Autodesk Inventor part; units mm, degrees
ref_plane "YZ Plane" through (0, 0, 0) normal (1, 0, 0) x (0, 1, 0)
ref_plane "XZ Plane" through (0, 0, 0) normal (0, 1, 0) x (-1, 0, 0)
ref_plane "XY Plane" through (0, 0, 0) normal (0, 0, 1) x (1, 0, 0)
sketch "Sketch1" plane through (0, 0, 0) normal (0, 1, 0) x (-1, 0, 0)
  circle A0 centre (-65.9389, 138.5386) radius 14
  circle A1 centre (-65.9389, 138.5386) radius 13.746
  circle A2 centre (-65.9389, 138.5386) radius 31.75
  point P0 (0, 0)
  dimension "d0" = 27.492
  dimension "d1" = 28
  dimension "d2" = 63.5
extrude "Extrusion1" add sketch "Sketch1" along normal blind 3.175 contours A0 | A1 | A2
sketch "Sketch2" plane through (65.9389, 0, 138.5386) normal (0, -1, 0) x (1, 0, 0)
  circle A0 centre (0, 0) radius 13.746
  point P0 (-65.9389, -138.5386)
  dimension "d5" = 27.492
extrude "Extrusion2" add sketch "Sketch2" along normal blind 38.1
sketch "Sketch3" plane through (65.9389, 0, 138.5386) normal (0, -1, 0) x (1, 0, 0)
  circle A0 centre (0, 23.8125) radius 2.1526
  circle A1 centre (20.6222, 11.9062) radius 2.1526
  circle A2 centre (20.6222, -11.9063) radius 2.1526
  circle A3 centre (0, -23.8125) radius 2.1526
  circle A4 centre (-20.6222, -11.9062) radius 2.1526
  circle A5 centre (-20.6222, 11.9063) radius 2.1526
  circle A6 centre (0, 23.8125) radius 1.8986
  circle A7 centre (20.6222, 11.9062) radius 1.8986
  circle A8 centre (20.6222, -11.9063) radius 1.8986
  circle A9 centre (-20.6222, -11.9062) radius 1.8986
  circle A10 centre (-20.6222, 11.9063) radius 1.8986
  circle A11 centre (0, -23.8125) radius 1.8986
  point P0 (-65.9389, -138.5386)
  dimension "d8" = 4.3053
  dimension "d9" = 3.7973
  dimension "d10" = 3.7973
  dimension "d11" = 3.7973
  dimension "d12" = 3.7973
  dimension "d13" = 3.7973
  dimension "d14" = 3.7973
extrude "Extrusion3" add sketch "Sketch3" along normal blind 12.7 contours A6 | A7 | A8 | A9 | A10 | A11
properties part number "5inCompliantWheelHub"
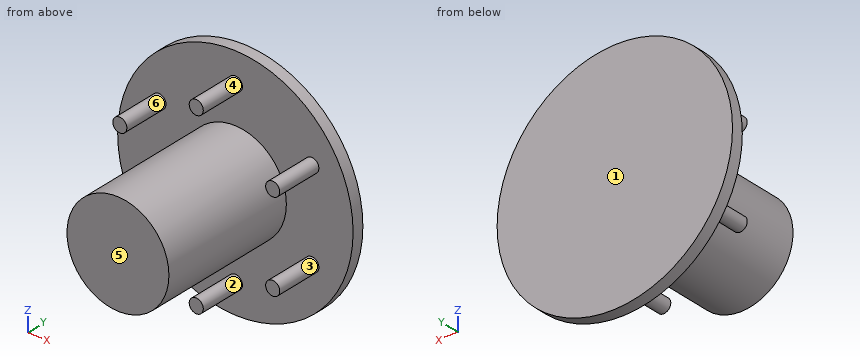
Can you work these out from the model? Positions are in its coordinate system, mm. Face numbers are marked on the shaded views. A direction names the side the tool comes from. Round coordinates to 2 decimals unless told otherwise and drop trailing zeros. Order: outer loops, then holes, each group sorted by start corner. A loop starts at its lowest first (then second) coordinate and runs counter-clockwise, first axis right, second up. Notation, with made-up numbers: (64, 35) -> (74, 35) arc R21 cw to (74, 45) -> close; hole circle Ø1 at (9, 78). An arc over 180 degrees is marked (long way). Return JSON: item names as keys, results as strings. Group by question number.
1. Will these pins go through, and if not, where does the flat tip stop? pin 1 (1.1 mm diameter, centred on x = 85.5, z = 151, fed in from -Y); pin 2 (1.5 mm diameter, centred on y = -15, z = 136, fed in from +X); pin 3 (2 mm diameter, centred on x = 79, z = 158, fed in from -Y).
2. We'd pull the mould along X, two halves only. Please class the marked faces 3, 4, 5 and 6: released by +X, released by -X, zero draft, split by the parting line, or undercut.
3. I need wall thicknesses on line 1 (Z direction, x = 45.5, y = -7.5); line 2 (Y direction, x = 68, z = 117.5) (3 decimals); line 3 (X direction, y = -9, z = 131). Which ranges of each line are inside material? Lowest first, please. Write a range as [from, to].
4. Which directions (+Z, -Z, +X, -X, +Y, -Y) give clear straight access to the entire face, cutting with the end or side of a thin tool? Please do the marked faces 1 and 2.
5. If we section it at C-C, the plane z = 144: Write out the boundary of the cut face in (x, y) (3 decimals), then the cut area to 3 significant figures.
6. If we section it at B-B, the plane x = 70: Write out the boundary of the cut face in (y, z) (3 decimals).
7. If we section it at D-D, the plane y = -22: Write out the boundary of the cut face in (x, z), then the cut area to 3 significant figures.
8. If we section it at A-A, the plane y = -3: Write out the boundary of the cut face in (x, z), then the cut area to 3 significant figures.
Output values:
{
 "1": {"pin 1": "y = -12.7", "pin 2": "x = 79.57", "pin 3": "y = 0"},
 "2": {"face 3": "undercut", "face 4": "split by the parting line", "face 5": "zero draft", "face 6": "undercut"},
 "3": {"line 1": "[124.74, 128.52], [148.56, 152.33]", "line 2": "[0, 3.175]", "line 3": "[54.44, 77.43]"},
 "4": {"face 1": "+Z, -Z, +X, -X, +Y", "face 2": "-Y"},
 "5": {"outline": "(34.662, 0) -> (53.324, 0) -> (53.324, -38.1) -> (78.553, -38.1) -> (78.553, 0) -> (97.216, 0) -> (97.216, 3.175) -> (34.662, 3.175) -> close", "area": "1,160 mm²"},
 "6": {"outline": "(-38.1, 125.406) -> (0, 125.406) -> (0, 107.049) -> (3.175, 107.049) -> (3.175, 170.028) -> (0, 170.028) -> (0, 151.671) -> (-38.1, 151.671) -> close"},
 "7": {"outline": "circle Ø27.49 at (65.94, 138.54)", "area": "594 mm²"},
 "8": {"outline": "circle Ø3.8 at (45.32, 126.63); circle Ø3.8 at (45.32, 150.44); circle Ø27.49 at (65.94, 138.54); circle Ø3.8 at (65.94, 114.73); circle Ø3.8 at (65.94, 162.35); circle Ø3.8 at (86.56, 126.63); circle Ø3.8 at (86.56, 150.44)", "area": "662 mm²"}
}
